The listing builds one solid part. Answer for the finished solid, in the listing's coordinates (mm). A direction names the side the tool comes from. Round coordinates to 2 decimals unless told otherwise and drop trailing zeros. Loops run counter-clockwise (first coordinate to the right, second up) from the corner with the lowest first, then second, coordinate; pieces in that order, holes last. Notation, with made-up numbers: M 29,68.25 L 68,68.25 A18 cw 68,103.25 Z; hole C 20,62.5 d6. An arc over 180 degrees is marked long. Answer as a JSON object with one key per item and string values.
```python
from build123d import *

# Parameters (mm, degrees)
SKETCH_R  = 1.5
PAD_DEPTH = 4


with BuildPart() as part:
    # Sketch → Pad (new body)
    with BuildSketch(Plane.XY):
        with BuildLine():
            ThreePointArc((13.615765, 96.742557), (1.659489, 113.901298), (-13.999945, 100.039225))
            ThreePointArc((-13.999945, 100.039225), (-11.293951, 49.378275), (-2.926476, -0.660106))
            ThreePointArc((-2.926476, -0.660106), (0.356119, -2.978788), (2.99961, 0.048367))
            ThreePointArc((13.615765, 96.742557), (5.2705, 48.728918), (2.99961, 0.048367))
        make_face()
        with Locations((0.848022, 108.256565)):
            Circle(SKETCH_R, mode=Mode.SUBTRACT)
        with Locations((-1.971907, 80.801)):
            Circle(SKETCH_R, mode=Mode.SUBTRACT)
        Polygon((-5.355573, 106.581629), (6.581629, 105.355573), (4.231688, 82.475936), (-7.705514, 83.701992), align=None, mode=Mode.SUBTRACT)
    extrude(amount=PAD_DEPTH)


solid = part.part
```
Item 1: The part is cut by section A-A (z = 1.95). Give the vertices of the cut face in (x, y), then the cut area to 3 significant figures.
Values follow:
{"outline": "M -14,100.04 A451.9 ccw -2.93,-0.66 A3 ccw 3,0.05 A388.64 cw 13.62,96.74 A14 ccw long Z; hole M -7.71,83.7 L 4.23,82.48 L 6.58,105.36 L -5.36,106.58 Z; hole C -1.97,80.8 d3; hole C 0.85,108.26 d3", "area": "1,720 mm^2"}
Item 2: The part is cut by section B-B (y = 21.5). Give the vertices of the cut face in (x, z).
Values follow:
{"outline": "M -7.35,0 L 3.25,0 L 3.25,4 L -7.35,4 Z"}
Item 3: Straight lines are drawn through the part: line 1 (X direction, y = 93, z = 2.8); line 2 (X direction, y = 92.5, z = 3.8); line 3 (X direction, y = 52, z = 2.6). For each, find the intervals that lie inside material, in ascending order.
Values follow:
{"line 1": "-13.96 to -6.75, 5.31 to 12.74", "line 2": "-13.96 to -6.8, 5.26 to 12.63", "line 3": "-11.57 to 5.64"}
Item 4: Flat-ended cylindrical pins translate along their axes: P1, Ø1, axis at y = 67.5, z = 3, coming from the +X side; P2, Ø1.8, axis at x = 0.85, y = 108.26, coming from the +Z side. Find the tip coordinate at first contact, or state that the pin passes through.
Values follow:
{"P1": "x = 7.88", "P2": "through"}
Item 5: Which of the six approach directions +Z, -Z, +X, -X, +Y, -Y give full straight-line access (tool end or side, diameter ignored) to faces 5 (the face through (0, 69, 4)), 6 (the face through (0.529, 105.977, 1.972))?
Values follow:
{"face 5": "+Z, +X, -X, +Y, -Y", "face 6": "+Z, -Z"}
Item 6: The part is cut by section C-C (y = 37.5). Give the vertices of the cut face in (x, z), then the cut area to 3 significant figures.
Values follow:
{"outline": "M -9.83,0 L 4.2,0 L 4.2,4 L -9.83,4 Z", "area": "56.1 mm^2"}
Item 7: Determine the mould class of faces 1 (the face through (-11.37, 50.08, 1.97)), 2 (the face through (-6.547, 94.982, 1.972)), 3 (the face through (0, 69, 0)), 4 (the face through (0, -3, 2)) for opening direction X: released by +X, released by -X, zero draft, split by the parting line, or undercut.
Values follow:
{"face 1": "released by -X", "face 2": "undercut", "face 3": "zero draft", "face 4": "split by the parting line"}
